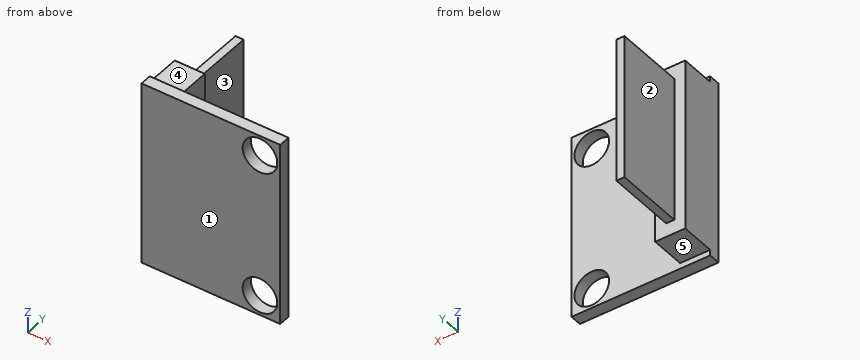
Autodesk Inventor part; units mm, degrees
ref_plane "YZ Plane" through (0, 0, 0) normal (1, 0, 0) x (0, 1, 0)
ref_plane "XZ Plane" through (0, 0, 0) normal (0, 1, 0) x (-1, 0, 0)
ref_plane "XY Plane" through (0, 0, 0) normal (0, 0, 1) x (1, 0, 0)
sketch "Sketch1" plane through (0, 0, 0) normal (0, 1, 0) x (-1, 0, 0)
  line L0 (-6, 8) -> (6, 8)
  line L1 (6, 8) -> (6, -8)
  line L2 (6, -8) -> (-6, -8)
  line L3 (-6, -8) -> (-6, 8)
  line L4 (-6, 8) -> (6, -8) construction
  line L5 (6, 8) -> (-6, -8) construction
  line L6 (-6, 8) -> (-4.25, 8)
  line L7 (-6, 6.25) -> (-6, 8)
  circle A0 centre (-4.25, 6.25) radius 1.5
  line L8 (0, 0) -> (-1.7804, 0)
  circle A1 centre (-4.25, -6.25) radius 1.5
  dimension "d0" = 12
  dimension "d1" = 16
  dimension "d4" = 3
  dimension "d7" = 1.75
extrude "Extrusion1" add sketch "Sketch1" along normal blind 1
sketch "Sketch2" plane through (0, 1, 0) normal (0, 1, 0) x (1, 0, 0)
  line L0 (-6, 8) -> (-6, -8)
  line L1 (-3.4, 7.5) -> (-6, 7.5)
  line L2 (-6, 7.5) -> (-6, -7.5)
  line L3 (-6, -7.5) -> (-3.4, -7.5)
  line L4 (-3.4, -7.5) -> (-3.4, 7.5)
  line L5 (-3.4, 7.5) -> (-6, -7.5) construction
  line L6 (-6, 7.5) -> (-3.4, -7.5) construction
  point P0 (0, 0)
  dimension "d9" = 2.6
  dimension "d10" = 15
extrude "Extrusion2" add sketch "Sketch2" along normal blind 3
sketch "Sketch3" plane through (0, 4, 0) normal (0, 1, 0) x (1, 0, 0)
  line L0 (-6, -7.5) -> (-6, -8)
  line L1 (-6, 7.5) -> (-3.4, 7.5)
  line L2 (-6, 7.5) -> (-6, -7.5)
  line L3 (-3.4, -7.5) -> (-3.4, 7.5)
  line L4 (-4.35, -6.3) -> (-5.05, -6.3)
  line L5 (-5.05, -6.3) -> (-5.05, 6.3)
  line L6 (-5.05, 6.3) -> (-4.35, 6.3)
  line L7 (-4.35, 6.3) -> (-4.35, -6.3)
  line L8 (-4.35, -6.3) -> (-5.05, 6.3) construction
  line L9 (-5.05, -6.3) -> (-4.35, 6.3) construction
  point P0 (0, 0)
  point P1 (-4.7, 0)
  dimension "d13" = 12.6
  dimension "d14" = 0.7
extrude "Extrusion3" add sketch "Sketch3" along normal blind 6
properties part number "SensorPresionHumedadTemp"
For this review, take the finished solid that the model builds, in its own axes (mm). Face numbers are marked on the shaded views. A direction names the side the tool comes from. Round coordinates to 2 decimals unless told otherwise and drop trailing zeros. Write each loop counter-clockwise with the first axis right and the second up, starting at its lowest first coordinate (ties: lowest second). Pieces come first, ordered by that corner, then holes. Notation, with made-up numbers: M 71,41.25 L 125,41.25 A30 ccw 125,73.25 Z; hole C 80.5,67.5 d4. An arc over 180 degrees is marked long. One line per item, written item: value. Start each with the question number.
(1) We need section D-D (x = -0.5). Give the boundary of the cut face in (y, z).
(2) The part is to be moulded in two halves that separate along Y. For the marked faces 1 and 2, say which applies: released by +Y, released by -Y, zero draft, split by the parting line, or undercut.
(3) We need section C-C (y = 2). Give the boundary of the cut face in (x, z).
(4) Machinability: for the marked faces 3, 4 and 5, which of the approach directions +Z, -Z, +X, -X, +Y, -Y give a long, thin tool a straight path to every point of the face, cutting with its end or side? Answer none if there is none.
(5) We need section A-A (z = 0.75). Give the boundary of the cut face in (x, y).
(6) We need section B-B (x = 4.25). Give the boundary of the cut face in (y, z).
(7) Insertion check: pin 1 (0.8 mm diameter, centred on x = -5, y = 7, fed in from +Z); pin 2 (2 mm diameter, centred on x = 1.5, z = -4.5, fed in from +Y); pin 3 (3 mm diameter, centred on x = -5, y = 3, fed in from -Z); pin 4 (2.5 mm diameter, centred on x = 4.25, z = 6.25, fed in from -Y). Each pin has a flat end and moves straight along its axis. Give the tip position at first contact, or say it passes through.
(8) Wall thickness on line 1 (Z direction, x = 4.25, y = 0.2); line 2 (Y direction, x = -1, z = 4); line 3 (X direction, y = 1.25, z = 2.5): over which ranges is each line inside the solid? List them lowest first.
Result:
1. outline: M 0,-8 L 1,-8 L 1,8 L 0,8 Z
2. face 1: released by -Y
2. face 2: zero draft
3. outline: M -6,-7.5 L -3.4,-7.5 L -3.4,7.5 L -6,7.5 Z
4. face 3: +Z, -Z, +X, +Y
4. face 4: +Z, +X, -X, +Y
4. face 5: -Z, +X, -X, +Y
5. outline: M -6,0 L 6,0 L 6,1 L -3.4,1 L -3.4,4 L -4.35,4 L -4.35,10 L -5.05,10 L -5.05,4 L -6,4 Z
6. outline: M 0,-8 L 1,-8 L 1,-7.75 L 0,-7.75 Z; M 0,-4.75 L 1,-4.75 L 1,4.75 L 0,4.75 Z; M 0,7.75 L 1,7.75 L 1,8 L 0,8 Z
7. pin 1: z = 6.3
7. pin 2: y = 1
7. pin 3: z = -7.5
7. pin 4: through
8. line 1: -8 to -7.75, -4.75 to 4.75, 7.75 to 8
8. line 2: 0 to 1
8. line 3: -6 to -3.4
